```python
from build123d import *

# Parameters (mm, degrees)
F0_R     = 152.4
F1_DEPTH = 254
F2_DEPTH = 127


with BuildPart() as f1:
    # F0 (on Front) → F1 (new body)
    with BuildSketch(Plane.XZ):
        with Locations((0, -51.59375)):
            Circle(F0_R)
        with BuildLine():
            ThreePointArc((-28.7373556529, 45.857388475), (-14.5176501359, 48.963685501), (0, 50.00625))
            ThreePointArc((0, 50.00625), (71.8420489686, 20.2482989686), (101.6, -51.59375))
            ThreePointArc((101.6, -51.59375), (-60.8393156835, -132.9641233995), (-28.7373556529, 45.857388475))
        make_face(mode=Mode.SUBTRACT)
        with BuildLine():
            Line((-28.7373556529, 45.857388475), (-25.5163285875, 43.1329727939))
            ThreePointArc((-25.5163285875, 43.1329727939), (-13.2129194743, 48.257842828), (0, 50.00625))
            ThreePointArc((0, 50.00625), (-14.5176501359, 48.963685501), (-28.7373556529, 45.857388475))
        make_face()
        with BuildLine():
            ThreePointArc((50.8, -0.79375), (-25.3417689572, -44.8214088762), (-25.5163285875, 43.1329727939))
            Line((-25.5163285875, 43.1329727939), (-28.7373556529, 45.857388475))
            ThreePointArc((-28.7373556529, 45.857388475), (-60.8393156835, -132.9641233995), (101.6, -51.59375))
            ThreePointArc((101.6, -51.59375), (71.8420489686, 20.2482989686), (0, 50.00625))
            ThreePointArc((0, 50.00625), (35.9210244843, 35.1272744843), (50.8, -0.79375))
        make_face()
    extrude(amount=F1_DEPTH)

    # F0 (on Front) → F2 (cut)
    with BuildSketch(Plane.XZ):
        with BuildLine():
            ThreePointArc((50.8, -0.79375), (-25.3417689572, -44.8214088762), (-25.5163285875, 43.1329727939))
            Line((-25.5163285875, 43.1329727939), (-28.7373556529, 45.857388475))
            ThreePointArc((-28.7373556529, 45.857388475), (-60.8393156835, -132.9641233995), (101.6, -51.59375))
            ThreePointArc((101.6, -51.59375), (71.8420489686, 20.2482989686), (0, 50.00625))
            ThreePointArc((0, 50.00625), (35.9210244843, 35.1272744843), (50.8, -0.79375))
        make_face()
    extrude(amount=F2_DEPTH, mode=Mode.SUBTRACT)


solid = f1.part
```
Could you check a few things on this model? Use its own coordinates, in mm. Coordinates: 2 decimals unless noted, no trailing zeros. Order: outer loops, then holes, each group sorted by start corner. A loop starts at its lowest first (then second) coordinate and runs counter-clockwise, first axis right, second up. Notation, with made-up numbers: M 87.5,-38 L 137.5,-38 A29 cw 137.5,-4 Z; hole C -19,84 d2. An arc over 180 degrees is marked long. Use a Markdown table: item, result. Add a question column.
Q1. I want a section at A-A on z = 11. List the corners of the cut face in (x, y) for me.
Q2. We'd pull the mould along X, two halves only. Please class faces 1 (the flat face through (-1, -127, -73)), 2 (the cylindrical face through (-33.04, -125.22, -200.37)), 3 (the flat face through (32, 0, -151)), 4 (the cylindrical face through (-11, -181.7, 48.8)): pulls with the +X half, pulls with the -X half, needs draft (parallel to the pull), parting line crosses it, or undercut.
Q3. I want a section at C-C on x = 65. List the corners of the cut face in (y, z) for me.
Q4. I'm going to push flat-ended pins straight in: pin 1 (12 mm diameter, centred on y = -144.5, z = -3, fed in from -X); pin 2 (3 mm diameter, centred on x = 84.5, y = -109, fed in from -Z); pin 3 (5 mm diameter, centred on y = -202.5, z = -143.5, fed in from -X). Where does each tip first touch, or does it pass through?
Q5. If I drill on L1, parallel to Z at x = 0, y = -203; L2, parallel to Z at x = 0, y = -65; L3, parallel to Y at x = 53.5, z = -101, over which ranges is the centre line in solid material (lowest first)?
Q6. I want a section at D-D on z = -66. List the corners of the cut face in (x, y) for me.
Q7. I want a section at B-B on y = -92. List the corners of the cut face in (x, z) for me, then the cut area to 3 significant figures.
Checked values:
| question | item | result |
|---|---|---|
| 1 | outline | M -138.95,-254 L -49.41,-254 L -49.41,-127 L -80.03,-127 L -80.03,0 L -138.95,0 Z; M 49.41,-254 L 138.95,-254 L 138.95,0 L 80.03,0 L 80.03,-127 L 49.41,-127 Z |
| 2 | face 1 | undercut |
| 2 | face 2 | parting line crosses it |
| 2 | face 3 | needs draft |
| 2 | face 4 | undercut |
| 3 | outline | M -254,-189.44 L 0,-189.44 L 0,-129.68 L -127,-129.68 L -127,26.49 L 0,26.49 L 0,86.25 L -254,86.25 Z |
| 4 | pin 1 | x = -146.33 |
| 4 | pin 2 | z = -179.41 |
| 4 | pin 3 | x = -123.42 |
| 5 | L1 | -203.99 to -51.59, 50.01 to 100.81 |
| 5 | L2 | -203.99 to -153.19, 50.01 to 100.81 |
| 5 | L3 | -254 to -127 |
| 6 | outline | M -151.72,-254 L 151.72,-254 L 151.72,0 L 100.57,0 L 100.57,-127 L -100.57,-127 L -100.57,0 L -151.72,0 Z |
| 7 | outline | C 0,-51.59 d304.8; hole M -28.74,45.86 A101.6 ccw long 0,50.01 A50.8 ccw -25.52,43.13 Z |
| 7 | area | 40,600 mm² |
